Design review of the part built by this model. Coordinates are the model's own, in mm. Coordinates: 2 decimals unless noted, no trailing zeros. Loops run counter-clockwise (first coordinate to the right, second up) from the corner with the lowest first, then second, coordinate; pieces in that order, holes last.
Q1. Wall thickness on probe 1 along Y at (x, z) = (171, 0.1); probe 2 along Y at (x, z) = (170, 0.75); probe 3 along X at (y, z) = (5, 0.7): over which ranges is each line inside the solid? List them lowest first.
Q2. Add section B-B on x = 171. Give the boundary of the cut face in (y, z), and give its area (3 significant figures).
Q3. For P1, Ø2.5, axis at x = 171, y = 5, coming from the +Z side, flat-tipped, find the tip position at first contact; note if it passes through.
Q4. Add section C-C on z = 2.4. Give the boundary of the cut face in (x, y), and give its area (3 significant figures).
Q5. Add section A-A on y = 15. Give the boundary of the cut face in (x, z).
```python
from build123d import *

# Parameters (mm, degrees)
SKIZZE1_W                       = 177
SKIZZE1_H                       = 20
AUFSATZ_LINEAR_AUSTRAGEN1_DEPTH = 3
SKIZZE3_R                       = 2
SCHNITT_LINEAR_AUSTRAGEN1_DEPTH = 8
FASE1_SIZE                      = 2.7
SKIZZE5_R                       = 2
SCHNITT_LINEAR_AUSTRAGEN2_DEPTH = 8
FASE2_SIZE                      = 2.7


with BuildPart() as part:
    # Skizze1 → Aufsatz-Linear austragen1 (new body)
    with BuildSketch(Plane.XY):
        with Locations((88.5, 10)):
            Rectangle(SKIZZE1_W, SKIZZE1_H)
    extrude(amount=AUFSATZ_LINEAR_AUSTRAGEN1_DEPTH)

    # Skizze3 → Schnitt-Linear austragen1 (cut)
    with BuildSketch(Plane.XY.offset(3)):
        with Locations((171, 5)):
            Circle(SKIZZE3_R)
    extrude(amount=-SCHNITT_LINEAR_AUSTRAGEN1_DEPTH, mode=Mode.SUBTRACT)

    # Fase1
    fase1_edges = [part.edges().sort_by_distance(p)[0] for p in [
        (169, 5, 3),
    ]]
    chamfer(fase1_edges, length=FASE1_SIZE)

    # Skizze5 → Schnitt-Linear austragen2 (cut)
    with BuildSketch(Plane.XY.offset(3)):
        with Locations((171, 15)):
            Circle(SKIZZE5_R)
    extrude(amount=-SCHNITT_LINEAR_AUSTRAGEN2_DEPTH, mode=Mode.SUBTRACT)

    # Fase2
    fase2_edges = [part.edges().sort_by_distance(p)[0] for p in [
        (169, 15, 3),
    ]]
    chamfer(fase2_edges, length=FASE2_SIZE)


solid = part.part
```
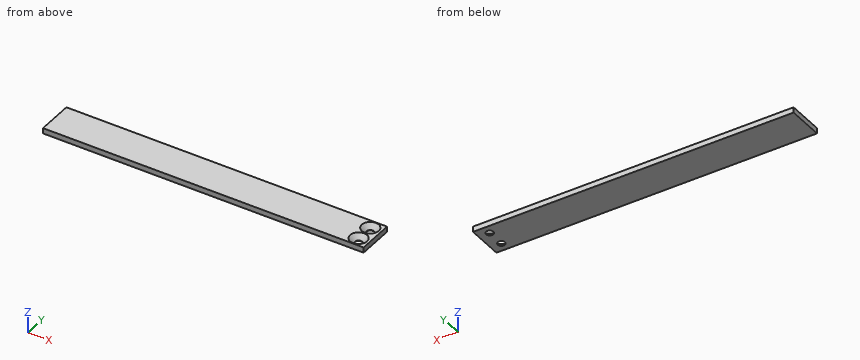
Entries:
1. probe 1: y = 0 to 3, 7 to 13, 17 to 20
1. probe 2: y = 0 to 2.76, 7.24 to 12.76, 17.24 to 20
1. probe 3: x = 0 to 168.6, 173.4 to 177
2. outline: (0, 0) - (3, 0) - (3, 0.3) - (0.3, 3) - (0, 3) - close; (7, 0) - (13, 0) - (13, 0.3) - (10.3, 3) - (9.7, 3) - (7, 0.3) - close; (17, 0) - (20, 0) - (20, 3) - (19.7, 3) - (17, 0.3) - close
2. area: 21.4 mm2
3. P1: passes through
4. outline: (0, 0) - (177, 0) - (177, 20) - (0, 20) - close; hole circle Ø8.2 at (171, 5); hole circle Ø8.2 at (171, 15)
4. area: 3,430 mm2
5. outline: (0, 0) - (169, 0) - (169, 0.3) - (166.3, 3) - (0, 3) - close; (173, 0) - (177, 0) - (177, 3) - (175.7, 3) - (173, 0.3) - close
